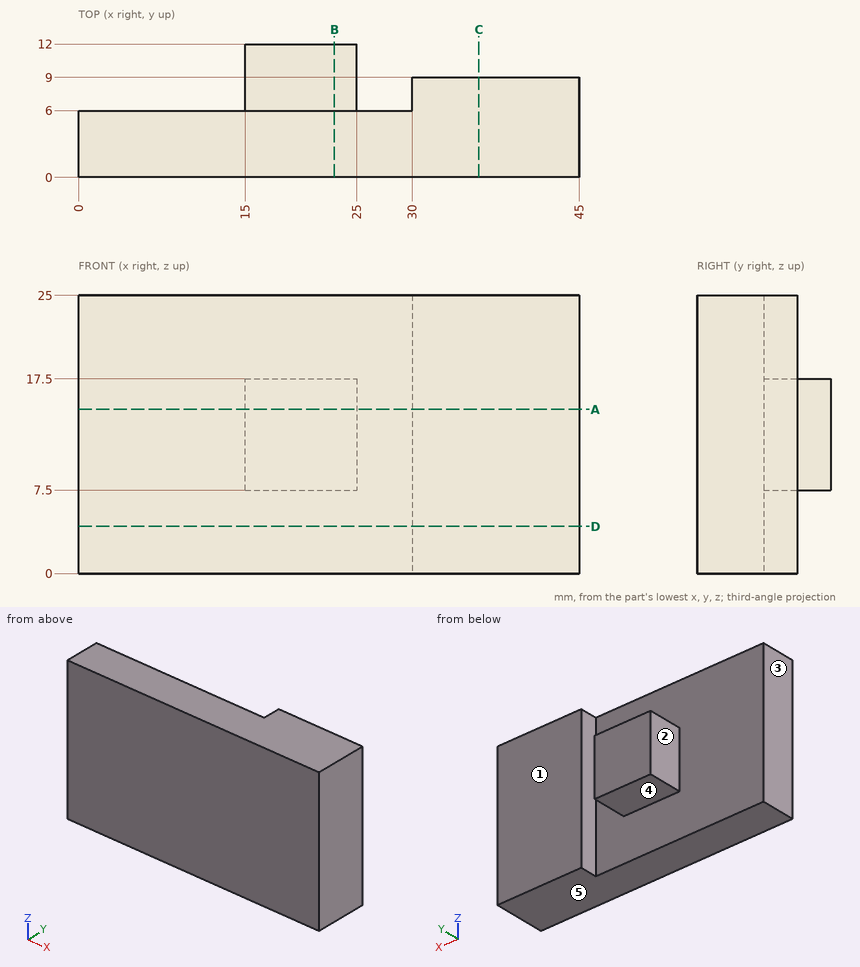
Here's the drawing with two shaded views (mm, measured from the low corner). I have some questions. A direction names the side the tool comes from. Round coordinates to 2 decimals unless told otherwise and drop trailing zeros. Loops run counter-clockwise (first coordinate to the right, second up) from the corner with the lowest first, then second, coordinate; pieces in that order, holes last. Notation, with made-up numbers: (82, 77.5) - (103, 77.5) arc R16 ccw to (103, 102.5) - close; hole circle Ø1 at (75.25, 80). An arc over 180 degrees is marked (long way). Use CSV: the item, a comma, the result in double quotes. Start each with the question number.
1) If we section it at B-B on x = 23: Write out the boundary of the cut face in (y, z).
2) Please list where these lines run through material, in increasing order: probe 1 along X at (y, z) = (8, 17); probe 2 along Y at (x, z) = (36.5, 18.5); probe 3 along Y at (x, z) = (29.5, 22.25). Write a range as [from, to].
3) If we section it at D-D on z = 4.25: Write out the boundary of the cut face in (x, y).
4) For the marked faces 1, 2, 3, 4 and 5, which set-ups out of +Z, -Z, +X, -X, +Y, -Y let a thin tool reach every point of the face, with its end or its side?
5) For pin 1 Ø5 at (y, z) = (9, 14.5) entering from -X; pin 2 Ø4 at (x, z) = (8.5, 15) entering from +Y; pin 3 Ø12 at (x, z) = (36, 8.5) entering from +Y, each with a flat end and sliding along its axis, tell me the tip position at first contact or that it passes through.
6) If we section it at A-A on z = 14.75: Write out the boundary of the cut face in (x, y), plus the area to 3 significant figures.
7) If we section it at C-C on x = 36: Write out the boundary of the cut face in (y, z), plus the area to 3 significant figures.
Geometry results:
1,outline,"(0, 0) - (6, 0) - (6, 7.5) - (12, 7.5) - (12, 17.5) - (6, 17.5) - (6, 25) - (0, 25) - close"
2,probe 1,"x = [15, 25], [30, 45]"
2,probe 2,"y = [0, 9]"
2,probe 3,"y = [0, 6]"
3,outline,"(0, 0) - (45, 0) - (45, 9) - (30, 9) - (30, 6) - (0, 6) - close"
4,face 1,"+Z, -Z, +X, +Y"
4,face 2,"+Z, -Z, -X, +Y"
4,face 3,"+Z, -Z, -X, +Y, -Y"
4,face 4,"-Z, -X, +Y"
4,face 5,"-Z, +X, -X, +Y, -Y"
5,pin 1,"stops at x = 15"
5,pin 2,"stops at y = 6"
5,pin 3,"stops at y = 9"
6,outline,"(0, 0) - (45, 0) - (45, 9) - (30, 9) - (30, 6) - (25, 6) - (25, 12) - (15, 12) - (15, 6) - (0, 6) - close"
6,area,"375 mm2"
7,outline,"(0, 0) - (9, 0) - (9, 25) - (0, 25) - close"
7,area,"225 mm2"
